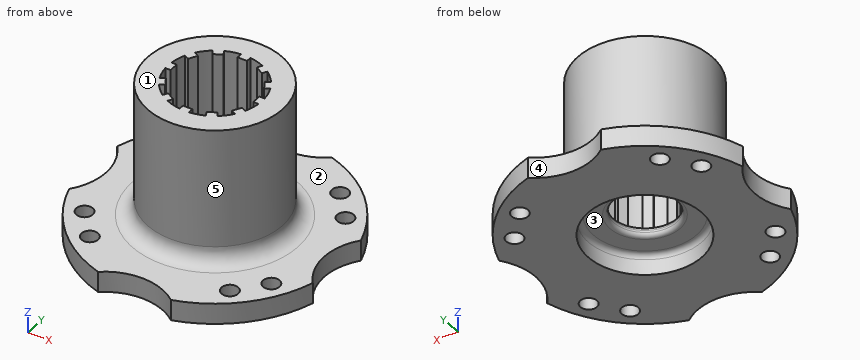
from build123d import *

# Parameters (mm, degrees)
SKETCH1_R           = 8
BOSS_EXTRUDE1_DEPTH = 20
BOSS_EXTRUDE2_START = 20
SKETCH1_3_R         = 65
BOSS_EXTRUDE2_DEPTH = 130
SKETCH2_R           = 55
SKETCH2_R_2         = 30
CUT_EXTRUDE1_DEPTH  = 20
BOSS_EXTRUDE3_START = -20
SKETCH2_2_R         = 55
SKETCH2_2_R_2       = 30
BOSS_EXTRUDE3_DEPTH = 10
FILLET1_R           = 15
FILLET2_R           = 4
FILLET3_R           = 5


with BuildPart() as part:
    # Sketch1 → Boss-Extrude1 (new body)
    with BuildSketch(Plane.XY):
        with BuildLine():
            ThreePointArc((117.165497838, -35.064741783), (104.8, 0), (117.165497838, 35.064741783))
            ThreePointArc((117.165497838, 35.064741783), (86.479159339, 86.479159339), (35.064741783, 117.165497838))
            ThreePointArc((35.064741783, 117.165497838), (0, 104.8), (-35.064741783, 117.165497838))
            ThreePointArc((-35.064741783, 117.165497838), (-86.479159339, 86.479159339), (-117.165497838, 35.064741783))
            ThreePointArc((-117.165497838, 35.064741783), (-104.8, 0), (-117.165497838, -35.064741783))
            ThreePointArc((-117.165497838, -35.064741783), (-86.479159339, -86.479159339), (-35.064741783, -117.165497838))
            ThreePointArc((-35.064741783, -117.165497838), (0, -104.8), (35.064741783, -117.165497838))
            ThreePointArc((35.064741783, -117.165497838), (86.479159339, -86.479159339), (117.165497838, -35.064741783))
        make_face()
        with Locations((-67.364141495, -80.281457639)):
            Circle(SKETCH1_R, mode=Mode.SUBTRACT)
        with Locations((-89.831133114, -53.975990251)):
            Circle(SKETCH1_R, mode=Mode.SUBTRACT)
        with Locations((67.364141495, -80.281457639)):
            Circle(SKETCH1_R, mode=Mode.SUBTRACT)
        with Locations((89.831133114, -53.975990251)):
            Circle(SKETCH1_R, mode=Mode.SUBTRACT)
        with Locations((-89.831133114, 53.975990251)):
            Circle(SKETCH1_R, mode=Mode.SUBTRACT)
        with Locations((-67.364141495, 80.281457639)):
            Circle(SKETCH1_R, mode=Mode.SUBTRACT)
        with Locations((89.831133114, 53.975990251)):
            Circle(SKETCH1_R, mode=Mode.SUBTRACT)
        with Locations((67.364141495, 80.281457639)):
            Circle(SKETCH1_R, mode=Mode.SUBTRACT)
        with BuildLine():
            Line((-4.5, 44.77443467), (-4.5, 39.77443467))
            Line((-4.5, 39.77443467), (4.5, 39.77443467))
            Line((4.5, 39.77443467), (4.5, 44.77443467))
            ThreePointArc((4.5, 44.77443467), (11.64685703, 43.466662183), (18.490103018, 41.025797864))
            Line((18.490103018, 41.025797864), (15.990103018, 36.695670845))
            Line((15.990103018, 36.695670845), (23.784331652, 32.195670845))
            Line((23.784331652, 32.195670845), (26.284331652, 36.525797864))
            ThreePointArc((26.284331652, 36.525797864), (31.819805153, 31.819805153), (36.525797864, 26.284331652))
            Line((36.525797864, 26.284331652), (32.195670845, 23.784331652))
            Line((32.195670845, 23.784331652), (36.695670845, 15.990103018))
            Line((36.695670845, 15.990103018), (41.025797864, 18.490103018))
            ThreePointArc((41.025797864, 18.490103018), (43.466662183, 11.64685703), (44.77443467, 4.5))
            Line((44.77443467, 4.5), (39.77443467, 4.5))
            Line((39.77443467, 4.5), (39.77443467, -4.5))
            Line((39.77443467, -4.5), (44.77443467, -4.5))
            ThreePointArc((44.77443467, -4.5), (43.466662183, -11.64685703), (41.025797864, -18.490103018))
            Line((41.025797864, -18.490103018), (36.695670845, -15.990103018))
            Line((36.695670845, -15.990103018), (32.195670845, -23.784331652))
            Line((32.195670845, -23.784331652), (36.525797864, -26.284331652))
            ThreePointArc((36.525797864, -26.284331652), (31.819805153, -31.819805153), (26.284331652, -36.525797864))
            Line((26.284331652, -36.525797864), (23.784331652, -32.195670845))
            Line((23.784331652, -32.195670845), (15.990103018, -36.695670845))
            Line((15.990103018, -36.695670845), (18.490103018, -41.025797864))
            ThreePointArc((18.490103018, -41.025797864), (11.64685703, -43.466662183), (4.5, -44.77443467))
            Line((4.5, -44.77443467), (4.5, -39.77443467))
            Line((4.5, -39.77443467), (-4.5, -39.77443467))
            Line((-4.5, -39.77443467), (-4.5, -44.77443467))
            ThreePointArc((-4.5, -44.77443467), (-11.64685703, -43.466662183), (-18.490103018, -41.025797864))
            Line((-18.490103018, -41.025797864), (-15.990103018, -36.695670845))
            Line((-15.990103018, -36.695670845), (-23.784331652, -32.195670845))
            Line((-23.784331652, -32.195670845), (-26.284331652, -36.525797864))
            ThreePointArc((-26.284331652, -36.525797864), (-31.819805153, -31.819805153), (-36.525797864, -26.284331652))
            Line((-36.525797864, -26.284331652), (-32.195670845, -23.784331652))
            Line((-32.195670845, -23.784331652), (-36.695670845, -15.990103018))
            Line((-36.695670845, -15.990103018), (-41.025797864, -18.490103018))
            ThreePointArc((-41.025797864, -18.490103018), (-43.466662183, -11.64685703), (-44.77443467, -4.5))
            Line((-44.77443467, -4.5), (-39.77443467, -4.5))
            Line((-39.77443467, -4.5), (-39.77443467, 4.5))
            Line((-39.77443467, 4.5), (-44.77443467, 4.5))
            ThreePointArc((-44.77443467, 4.5), (-43.466662183, 11.64685703), (-41.025797864, 18.490103018))
            Line((-41.025797864, 18.490103018), (-36.695670845, 15.990103018))
            Line((-36.695670845, 15.990103018), (-32.195670845, 23.784331652))
            Line((-32.195670845, 23.784331652), (-36.525797864, 26.284331652))
            ThreePointArc((-36.525797864, 26.284331652), (-31.819805153, 31.819805153), (-26.284331652, 36.525797864))
            Line((-26.284331652, 36.525797864), (-23.784331652, 32.195670845))
            Line((-23.784331652, 32.195670845), (-15.990103018, 36.695670845))
            Line((-15.990103018, 36.695670845), (-18.490103018, 41.025797864))
            ThreePointArc((-18.490103018, 41.025797864), (-11.64685703, 43.466662183), (-4.5, 44.77443467))
        make_face(mode=Mode.SUBTRACT)
    extrude(amount=BOSS_EXTRUDE1_DEPTH)

    # Sketch1<3> → Boss-Extrude2 (add)
    with BuildSketch(Plane.XY.offset(BOSS_EXTRUDE2_START)):
        Circle(SKETCH1_3_R)
        with BuildLine():
            Line((-4.5, 44.77443467), (-4.5, 39.77443467))
            Line((-4.5, 39.77443467), (4.5, 39.77443467))
            Line((4.5, 39.77443467), (4.5, 44.77443467))
            ThreePointArc((4.5, 44.77443467), (11.64685703, 43.466662183), (18.490103018, 41.025797864))
            Line((18.490103018, 41.025797864), (15.990103018, 36.695670845))
            Line((15.990103018, 36.695670845), (23.784331652, 32.195670845))
            Line((23.784331652, 32.195670845), (26.284331652, 36.525797864))
            ThreePointArc((26.284331652, 36.525797864), (31.819805153, 31.819805153), (36.525797864, 26.284331652))
            Line((36.525797864, 26.284331652), (32.195670845, 23.784331652))
            Line((32.195670845, 23.784331652), (36.695670845, 15.990103018))
            Line((36.695670845, 15.990103018), (41.025797864, 18.490103018))
            ThreePointArc((41.025797864, 18.490103018), (43.466662183, 11.64685703), (44.77443467, 4.5))
            Line((44.77443467, 4.5), (39.77443467, 4.5))
            Line((39.77443467, 4.5), (39.77443467, -4.5))
            Line((39.77443467, -4.5), (44.77443467, -4.5))
            ThreePointArc((44.77443467, -4.5), (43.466662183, -11.64685703), (41.025797864, -18.490103018))
            Line((41.025797864, -18.490103018), (36.695670845, -15.990103018))
            Line((36.695670845, -15.990103018), (32.195670845, -23.784331652))
            Line((32.195670845, -23.784331652), (36.525797864, -26.284331652))
            ThreePointArc((36.525797864, -26.284331652), (31.819805153, -31.819805153), (26.284331652, -36.525797864))
            Line((26.284331652, -36.525797864), (23.784331652, -32.195670845))
            Line((23.784331652, -32.195670845), (15.990103018, -36.695670845))
            Line((15.990103018, -36.695670845), (18.490103018, -41.025797864))
            ThreePointArc((18.490103018, -41.025797864), (11.64685703, -43.466662183), (4.5, -44.77443467))
            Line((4.5, -44.77443467), (4.5, -39.77443467))
            Line((4.5, -39.77443467), (-4.5, -39.77443467))
            Line((-4.5, -39.77443467), (-4.5, -44.77443467))
            ThreePointArc((-4.5, -44.77443467), (-11.64685703, -43.466662183), (-18.490103018, -41.025797864))
            Line((-18.490103018, -41.025797864), (-15.990103018, -36.695670845))
            Line((-15.990103018, -36.695670845), (-23.784331652, -32.195670845))
            Line((-23.784331652, -32.195670845), (-26.284331652, -36.525797864))
            ThreePointArc((-26.284331652, -36.525797864), (-31.819805153, -31.819805153), (-36.525797864, -26.284331652))
            Line((-36.525797864, -26.284331652), (-32.195670845, -23.784331652))
            Line((-32.195670845, -23.784331652), (-36.695670845, -15.990103018))
            Line((-36.695670845, -15.990103018), (-41.025797864, -18.490103018))
            ThreePointArc((-41.025797864, -18.490103018), (-43.466662183, -11.64685703), (-44.77443467, -4.5))
            Line((-44.77443467, -4.5), (-39.77443467, -4.5))
            Line((-39.77443467, -4.5), (-39.77443467, 4.5))
            Line((-39.77443467, 4.5), (-44.77443467, 4.5))
            ThreePointArc((-44.77443467, 4.5), (-43.466662183, 11.64685703), (-41.025797864, 18.490103018))
            Line((-41.025797864, 18.490103018), (-36.695670845, 15.990103018))
            Line((-36.695670845, 15.990103018), (-32.195670845, 23.784331652))
            Line((-32.195670845, 23.784331652), (-36.525797864, 26.284331652))
            ThreePointArc((-36.525797864, 26.284331652), (-31.819805153, 31.819805153), (-26.284331652, 36.525797864))
            Line((-26.284331652, 36.525797864), (-23.784331652, 32.195670845))
            Line((-23.784331652, 32.195670845), (-15.990103018, 36.695670845))
            Line((-15.990103018, 36.695670845), (-18.490103018, 41.025797864))
            ThreePointArc((-18.490103018, 41.025797864), (-11.64685703, 43.466662183), (-4.5, 44.77443467))
        make_face(mode=Mode.SUBTRACT)
    extrude(amount=BOSS_EXTRUDE2_DEPTH)

    # Sketch2 → Cut-Extrude1 (cut)
    with BuildSketch(Plane(origin=(0, 0, 0), x_dir=(-1, 0, 0), z_dir=(0, 0, -1))):
        Circle(SKETCH2_R)
        Circle(SKETCH2_R_2, mode=Mode.SUBTRACT)
    extrude(amount=-CUT_EXTRUDE1_DEPTH, mode=Mode.SUBTRACT)

    # Sketch2<2> → Boss-Extrude3 (add)
    with BuildSketch(Plane(origin=(0, 0, 0), x_dir=(-1, 0, 0), z_dir=(0, 0, -1)).offset(BOSS_EXTRUDE3_START)):
        Circle(SKETCH2_2_R)
        Circle(SKETCH2_2_R_2, mode=Mode.SUBTRACT)
    extrude(amount=-BOSS_EXTRUDE3_DEPTH)

    # Fillet1
    fillet1_edges = [part.edges().sort_by_distance(p)[0] for p in [
        (-65, 0, 20),
    ]]
    fillet(fillet1_edges, radius=FILLET1_R)

    # Fillet2
    fillet2_edges = [part.edges().sort_by_distance(p)[0] for p in [
        (30, 0, 30),
        (30, 0, 20),
    ]]
    fillet(fillet2_edges, radius=FILLET2_R)

    # Fillet3
    fillet3_edges = [part.edges().sort_by_distance(p)[0] for p in [
        (55, 0, 20),
    ]]
    fillet(fillet3_edges, radius=FILLET3_R)


solid = part.part
The listing builds one solid part. Answer for the finished solid, in the listing's coordinates (mm). Face numbers are marked on the shaded views. A direction names the side the tool comes from. Give positions to 0.01 mm unless a question says otherwise; leave off trailing zeros. Write each loop counter-clockwise with the first axis right and the second up, starting at its lowest first coordinate (ties: lowest second). Pieces come first, ordered by that corner, then holes.
Item 1: Flat-ended cylindrical pins translate along their axes: P1, Ø8, axis at y = 45, z = 125, coming from the -X side; P2, Ø13, axis at x = -89.83, y = 53.98, coming from the +Z side; P3, Ø10, axis at x = 0, z = 61.5, coming from the -Y side; P4, Ø5.5, axis at x = -42, z = 84.5, coming from the +Y side. Find the tip coordinate at first contact, or state that the pin passes through.
Item 2: Find the intervals of material crossed by line 1 along Z through (x, y) = (99.5, -48); line 2 along Z through (x, y) = (27.5, -30); line 3 along Y through (x, z) = (-30, 56), in increasing order.
Item 3: Determine the mould class of the marked faces 3, 4 and 5 for opening direction Y: released by +Y, released by -Y, zero draft, split by the parting line, or undercut.
Item 4: Section C-C, the plane x = 94 is taken. Write down the section's boundary in (y, z), plus the area to 3 significant figures.
Item 5: Which of the six approach directions +Z, -Z, +X, -X, +Y, -Y give full straight-line access (tool end or side, diameter ignored) to the marked faces 1 and 2?
Item 6: Section A-A, the plane y = 0 is taken. Write down the section's boundary in (x, z), plus the area to 3 significant figures.
Item 7: Section D-D, the plane x = -101 is taken. Write down the section's boundary in (y, z), plus the area to 3 significant figures.
Completed:
1. P1: stops at x = -50.44
1. P2: passes through
1. P3: stops at y = -65
1. P4: stops at y = 51.81
2. line 1: z = 0 to 20
2. line 2: z = 20 to 30
2. line 3: y = -57.66 to -33.54, 33.54 to 57.66
3. face 3: undercut
3. face 4: released by +Y
3. face 5: split by the parting line
4. outline: (-78.24, 0) - (-60.8, 0) - (-60.8, 20) - (-78.24, 20) - close; (-47.15, 0) - (47.15, 0) - (47.15, 20) - (-47.15, 20) - close; (60.8, 0) - (78.24, 0) - (78.24, 20) - (60.8, 20) - close
4. area: 2,580 mm2
5. face 1: +Z, +X, -X, +Y, -Y
5. face 2: +Z
6. outline: (-104.8, 0) - (-55, 0) - (-55, 15) arc R5 cw to (-50, 20) - (-34, 20) arc R4 ccw to (-30, 24) - (-30, 26) arc R4 ccw to (-34, 30) - (-39.77, 30) - (-39.77, 150) - (-65, 150) - (-65, 35) arc R15 cw to (-80, 20) - (-104.8, 20) - close; (30, 24) arc R4 ccw to (34, 20) - (50, 20) arc R5 cw to (55, 15) - (55, 0) - (104.8, 0) - (104.8, 20) - (80, 20) arc R15 cw to (65, 35) - (65, 150) - (39.77, 150) - (39.77, 30) - (34, 30) arc R4 ccw to (30, 26) - close
6. area: 8,840 mm2
7. outline: (-68.97, 0) - (68.97, 0) - (68.97, 20) - (-68.97, 20) - close
7. area: 2,760 mm2
